```python
from build123d import *

# Parameters (mm, degrees)
F0_W           = 27
F0_H           = 40
F1_DEPTH       = 32
F3_D           = 3.3
F3_CBORE_D     = 6.5
F3_CBORE_DEPTH = 3
F4_D           = 5


with BuildPart() as f1:
    # F0 (on Top) → F1 (new body)
    with BuildSketch(Plane.XY):
        with Locations((-23.3004702032, -43.8329163194)):
            Rectangle(F0_W, F0_H)
    extrude(amount=F1_DEPTH)

    # F3 (through all)
    with Locations(Plane.XY.offset(32)):
        with Locations((-33.3004702032, -33.8329163194), (-13.3004702032, -33.8329163194), (-13.3004702032, -53.8329163194), (-33.3004702032, -53.8329163194)):
            CounterBoreHole(F3_D / 2, F3_CBORE_D / 2, F3_CBORE_DEPTH)

    # F4 (through all)
    with Locations(Plane.XY.offset(32)):
        with Locations((-23.3004702032, -28.8329163194), (-23.3004702032, -58.8329163194)):
            Hole(F4_D / 2)


solid = f1.part
```
The model under review builds one solid part; all positions refer to its coordinate system, in mm. A direction names the side the tool comes from. Round coordinates to 2 decimals unless told otherwise and drop trailing zeros. Loops run counter-clockwise (first coordinate to the right, second up) from the corner with the lowest first, then second, coordinate; pieces in that order, holes last. Notation, with made-up numbers: (79.25, 26) - (86.25, 26) arc R22 ccw to (86.25, 42) - close; hole circle Ø6 at (-37, -40). An arc over 180 degrees is marked (long way). Use a Markdown table: item, result. Add a question column.
Q1. Add section B-B (x = -13.25). State the section outline as (y, z) points, plus the area to 3 significant figures.
Q2. Add section A-A (y = -28). State the section outline as (x, z) points.
Q3. The part is to be moulded in two halves that separate along X. For faces 3 (the face through (-23, -44, 32)), 4 (the face through (-36.8, -44, 16)), 5 (the face through (-35, -53, 29)), say which applies: pulls with the +X half, pulls with the -X half, needs draft (parallel to the pull), parting line crosses it, or undercut.
Q4. Machinability: for faces 1 (the face through (-34.825, -54.465, 14.297)), 2 (the face through (-13.72, -30.61, 30.52)), which of the approach directions +Z, -Z, +X, -X, +Y, -Y give a long, thin tool a straight path to every point of the face, cutting with its end or side? Answer none if there is none.
Q5. Add section D-D (y = -35). State the section outline as (x, z) points.
Q6. For probe 1 along X at (y, z) = (-34, 3); probe 2 along Y at (x, z) = (-23.75, 26); probe 3 along X at (y, z) = (-30, 12), list the stretches that pass through material, from the lowest coordinate up.
Q7. Add section C-C (z = 24). State the section outline as (x, y) points.
Q8. Insertion check: pin 1 Ø8 at (x, y) = (-23.3, -58.83) entering from -Z; pin 2 Ø2 at (x, y) = (-14, -52.5) entering from +Z. Each pin has a flat end and moves straight along its axis. Give the tip position at first contact, or say it passes through.
Worked answers:
| question | item | result |
|---|---|---|
| 1 | outline | (-63.83, 0) - (-55.48, 0) - (-55.48, 29) - (-57.08, 29) - (-57.08, 32) - (-63.83, 32) - close; (-52.18, 0) - (-35.48, 0) - (-35.48, 29) - (-37.08, 29) - (-37.08, 32) - (-50.58, 32) - (-50.58, 29) - (-52.18, 29) - close; (-32.18, 0) - (-23.83, 0) - (-23.83, 32) - (-30.58, 32) - (-30.58, 29) - (-32.18, 29) - close |
| 1 | area | 1,050 mm² |
| 2 | outline | (-36.8, 0) - (-25.66, 0) - (-25.66, 32) - (-36.8, 32) - close; (-20.94, 0) - (-9.8, 0) - (-9.8, 32) - (-20.94, 32) - close |
| 3 | face 3 | needs draft |
| 3 | face 4 | pulls with the -X half |
| 3 | face 5 | undercut |
| 4 | face 1 | +Z, -Z |
| 4 | face 2 | +Z |
| 5 | outline | (-36.8, 0) - (-34.47, 0) - (-34.47, 29) - (-36.33, 29) - (-36.33, 32) - (-36.8, 32) - close; (-32.13, 0) - (-14.47, 0) - (-14.47, 29) - (-16.33, 29) - (-16.33, 32) - (-30.27, 32) - (-30.27, 29) - (-32.13, 29) - close; (-12.13, 0) - (-9.8, 0) - (-9.8, 32) - (-10.27, 32) - (-10.27, 29) - (-12.13, 29) - close |
| 6 | probe 1 | -36.8 to -34.94, -31.66 to -14.94, -11.66 to -9.8 |
| 6 | probe 2 | -63.83 to -61.29, -56.37 to -31.29, -26.37 to -23.83 |
| 6 | probe 3 | -36.8 to -25.51, -21.09 to -9.8 |
| 7 | outline | (-36.8, -63.83) - (-9.8, -63.83) - (-9.8, -23.83) - (-36.8, -23.83) - close; hole circle Ø3.3 at (-33.3, -53.83); hole circle Ø3.3 at (-33.3, -33.83); hole circle Ø5 at (-23.3, -58.83); hole circle Ø5 at (-23.3, -28.83); hole circle Ø3.3 at (-13.3, -53.83); hole circle Ø3.3 at (-13.3, -33.83) |
| 8 | pin 1 | z = 0 |
| 8 | pin 2 | z = 29 |
